from build123d import *

# Parameters (mm, degrees)
SKETCH1_W                          = 609.6
SKETCH1_H                          = 406.4
BOSS_EXTRUDE1_DEPTH                = 4.7625
F_10_CLEARANCE_HOLE1_D             = 4.9784
F_10_CLEARANCE_HOLE1_DEPTH         = 10.16
F_10_CLEARANCE_HOLE1_TIP           = 1.495662253
F_6_CLEARANCE_HOLE1_D              = 3.6576
F_6_CLEARANCE_HOLE1_DEPTH          = 10.16
F_6_CLEARANCE_HOLE1_TIP            = 1.0988539
F_10_CLEARANCE_HOLE2_D             = 4.9784
F_10_CLEARANCE_HOLE2_DEPTH         = 10.16
F_10_CLEARANCE_HOLE2_TIP           = 1.495662253
CUT_EXTRUDE6_DEPTH                 = 5.7625
F_3_16_0_1875_DIAMETER_HOLE1_D     = 4.7625
F_3_16_0_1875_DIAMETER_HOLE1_DEPTH = 10.16
F_3_16_0_1875_DIAMETER_HOLE1_TIP   = 1.430799349


with BuildPart() as part:
    # Sketch1 → Boss-Extrude1 (new body)
    with BuildSketch(Plane.XY):
        with Locations((304.8, 203.2)):
            Rectangle(SKETCH1_W, SKETCH1_H)
    extrude(amount=BOSS_EXTRUDE1_DEPTH)

    # #10 Clearance Hole1
    with Locations(Plane.XY.offset(4.7625)):
        with Locations((393.7, 12.7), (304.8, 203.2), (596.9, 393.7), (12.7, 12.7), (12.7, 393.7), (596.9, 12.7), (304.8, 330.2), (304.8, 76.2)):
            Hole(F_10_CLEARANCE_HOLE1_D / 2, depth=F_10_CLEARANCE_HOLE1_DEPTH)
            with Locations((0, 0, -(F_10_CLEARANCE_HOLE1_DEPTH + F_10_CLEARANCE_HOLE1_TIP / 2))):  # 118° drill point
                Cone(0, F_10_CLEARANCE_HOLE1_D / 2, F_10_CLEARANCE_HOLE1_TIP, mode=Mode.SUBTRACT)

    # #6 Clearance Hole1
    with Locations(Plane.XY.offset(4.7625)):
        with Locations((153.8, 325.397045256), (115.7, 259.405909488), (77.6, 325.397045256), (178.748637136, 241.986495315), (365.913011093, 214.603454564), (378.514626904, 53.804869065), (229.881403774, 20.131066458), (87.511505802, 390.539377284), (106.048, 360.365035489), (125.352, 360.365035489), (143.888494198, 390.539377284)):
            Hole(F_6_CLEARANCE_HOLE1_D / 2, depth=F_6_CLEARANCE_HOLE1_DEPTH)
            with Locations((0, 0, -(F_6_CLEARANCE_HOLE1_DEPTH + F_6_CLEARANCE_HOLE1_TIP / 2))):  # 118° drill point
                Cone(0, F_6_CLEARANCE_HOLE1_D / 2, F_6_CLEARANCE_HOLE1_TIP, mode=Mode.SUBTRACT)

    # #10 Clearance Hole2
    with Locations(Plane.XY.offset(4.7625)):
        with Locations((165.89375, 132.55625), (115.09375, 132.55625)):
            Hole(F_10_CLEARANCE_HOLE2_D / 2, depth=F_10_CLEARANCE_HOLE2_DEPTH)
            with Locations((0, 0, -(F_10_CLEARANCE_HOLE2_DEPTH + F_10_CLEARANCE_HOLE2_TIP / 2))):  # 118° drill point
                Cone(0, F_10_CLEARANCE_HOLE2_D / 2, F_10_CLEARANCE_HOLE2_TIP, mode=Mode.SUBTRACT)

    # Sketch14 → Cut-Extrude6 (cut, through all)
    with BuildSketch(Plane.XY):
        with BuildLine():
            Line((609.6, 315.642514433), (609.6, 0))
            Line((609.6, 0), (432.195867807, 0))
            add(Edge.make_bspline(
                [(409.29659152, 170.617944662), (389.336707443, 111.226571114), (396.96980279, 54.353932563), (432.195867807, 0)],
                knots=[0.116936562, 0.116936562, 0.116936562, 0.116936562, 1, 1, 1, 1], degree=3))
            add(Edge.make_bspline(
                [(418.07234083, 177.13057308), (410.929678592, 177.953538089), (409.29659152, 170.617944662)],
                knots=[0, 0, 0, 1, 1, 1], degree=2))
            ThreePointArc((418.07234083, 177.13057308), (435.035932656, 180.354053738), (440.45974614, 196.747238983))
            Line((440.45974614, 196.747238983), (435.086955617, 221.682561203))
            add(Edge.make_bspline(
                [(435.086955617, 221.682561203), (465.243862883, 294.790369183), (498.032190497, 320.641169761), (609.6, 315.642514433)],
                knots=[0.107898544, 0.107898544, 0.107898544, 0.107898544, 1, 1, 1, 1], degree=3))
        make_face()
    extrude(amount=CUT_EXTRUDE6_DEPTH, mode=Mode.SUBTRACT)

    # 3/16 (0.1875) Diameter Hole1
    with Locations(Plane.XY.offset(4.7625)):
        with Locations((127.2, 314.9), (127.2, 291.9), (104.2, 291.9), (104.2, 314.9)):
            Hole(F_3_16_0_1875_DIAMETER_HOLE1_D / 2, depth=F_3_16_0_1875_DIAMETER_HOLE1_DEPTH)
            with Locations((0, 0, -(F_3_16_0_1875_DIAMETER_HOLE1_DEPTH + F_3_16_0_1875_DIAMETER_HOLE1_TIP / 2))):  # 118° drill point
                Cone(0, F_3_16_0_1875_DIAMETER_HOLE1_D / 2, F_3_16_0_1875_DIAMETER_HOLE1_TIP, mode=Mode.SUBTRACT)


solid = part.part
Part model, mm, in its own coordinate system. Coordinates: 2 decimals unless noted, no trailing zeros. Put each result on its own line as item: value.
1. Band-saw the part on A-A (z = 1.85). Give the number of separate pieces and of enclosed holes in the cut face, then the cut area to 3 significant figures.
Final values:
separate pieces: 1
enclosed holes: 24
area: 191,000 mm²
2. Flat gauge pin, fed straight in: pin 1 Ø6.5 at (x, y) = (165.89, 132.56) entering from -Z. Where does the tip first touch, or does it go through?
Final values:
pin 1: stops at z = 0
3. Probe line 1 along Y through (x, z) = (304.8, 2.95); line 2 along X through (y, z) = (361, 1.6); line 3 along Y through (x, z) = (127, 2.4). List the from-to ranges inside material, lowest first. Write a range as [from, to].
Final values:
line 1: y = [0, 73.71], [78.69, 200.71], [205.69, 327.71], [332.69, 406.4]
line 2: x = [0, 104.33], [107.76, 123.64], [127.07, 609.6]
line 3: y = [0, 289.53], [294.27, 312.53], [317.27, 359.57], [361.16, 406.4]
4. Two-plate mould, pull along Y, no slides. Class faces 1 (the flat face through (233, 206, 0)), 2 (the cylindrical face through (434.844, 180.188, 2.348)): +Y half, -Y half, draft (parallel to the pull), parting line (faces both ways), or undercut.
Final values:
face 1: draft
face 2: undercut
